The model under review builds one solid part; all positions refer to its coordinate system, in mm. Round coordinates to 2 decimals unless told otherwise and drop trailing zeros. Order: outer loops, then holes, each group sorted by start corner. A loop starts at its lowest first (then second) coordinate and runs counter-clockwise, first axis right, second up.
```python
from build123d import *

# Parameters (mm, degrees)
AILERON_DEPTH           = 482.696053238
SKETCH2_R               = 2.75
CUT_EXTRUDE2_DEPTH      = 483.696053238
CUT_EXTRUDE2_DEPTH_BACK = 484.024800506


with BuildPart() as part:
    # aileron_root → aileron (new body, symmetric, along a direction that is not the sketch's normal)
    with BuildSketch(Plane(origin=(0, 0, 0), x_dir=(0, 0, -1), z_dir=(1, 0, 0))):
        Polygon((-80, -10.492874398), (-80, 10.492874398), (0, 0), align=None)
    extrude(amount=AILERON_DEPTH, dir=(0.999991557, 0, 0.004109341), both=True)

    # Sketch2 → Cut-Extrude2 (cut, two sides)
    with BuildSketch(Plane(origin=(0, 0, 0), x_dir=(-0.004109341, 0, 0.999991557), z_dir=(-0.999991557, 0, -0.004109341))) as cut_extrude2_sk:
        with Locations((60, 0)):
            Circle(SKETCH2_R)
        Polygon((78.99932453, 0), (68.506450132, -10.492874398), (79.99932453, -10.492874398), (79.99932453, 10.492874398), (68.506450132, 10.492874398), align=None)
    extrude(amount=CUT_EXTRUDE2_DEPTH, mode=Mode.SUBTRACT)
    extrude(cut_extrude2_sk.sketch, amount=-CUT_EXTRUDE2_DEPTH_BACK, mode=Mode.SUBTRACT)


solid = part.part
```
(1) Insertion check: pin 1 (2 mm diameter, centred on x = 110.5, z = 45.5, fed in from +Y); pin 2 (10 mm diameter, centred on x = -339, z = 22.5, fed in from +Y); pin 3 (6 mm diameter, centred on x = -118, y = -6, fed in from +Z). Each pin has a flat end and moves straight along its axis. Give the tip position at first contact, or say it passes through.
Data:
pin 1: stops at y = 6.04
pin 2: stops at y = 3.79
pin 3: stops at z = 75.52
(2) Consider section A-A (z = 18). Write out the cut boundary in (x, y).
Data:
outline: (-482.69, -2.62) - (482.69, -2.1) - (482.69, 2.1) - (-482.69, 2.62) - close
(3) To check wall thickness, follow probe 1 along Y at (x, z) = (14, 58.5); probe 2 along Y at (x, z) = (234, 2); probe 3 along Y at (x, z) = (92, 17). State the ranges of each line that lie inside material, in increasing order.
Data:
probe 1: y = -7.67 to -2.27, 2.27 to 7.67
probe 2: y = -0.14 to 0.14
probe 3: y = -2.18 to 2.18
